Geometry: final body of the model. Coordinates: model frame, mm. A direction names the side the tool comes from. Give positions to 0.01 mm unless a question says otherwise; leave off trailing zeros. Write each loop counter-clockwise with the first axis right and the second up, starting at its lowest first coordinate (ties: lowest second). Pieces come first, ordered by that corner, then holes. Notation, with made-up numbers: M -1.5,-14.75 L 33.5,-14.75 A17 ccw 33.5,17.25 Z; hole C 71.25,2 d10. An arc over 180 degrees is marked long. Use a Markdown table: item, result. Add a question column.
(1) Cut plane C-C (z = 20). Output: boundary loops of the cut face in (x, y) (3 decimals), plus the area to 3 significant figures.
(2) Cut plane A-A (y = -39.5). Output: boundary loops of the cut face in (x, z) (3 decimals).
(3) Cut plane D-D (z = 63). Output: boundary loops of the cut face in (x, y) (3 decimals), plus the area to 3 significant figures.
(4) Material intervals for L1, parallel to X at y = -28.5, z = 153 (3 decimals); L2, parallel to Y at x = -20.25, z = 102.5 (3 decimals); L3, parallel to Y at x = -13.5, z = 16.5 (3 decimals), sorted ascending.
(5) Reachability of faces 1 (the flat face through (0, -20, 100)), 2 (the flat face through (-22.225, -26, 100)) from +Z, -Z, +X, -X, +Y, -Y: full face, straight path, thin tool, end or side. Return the list, or none.
(6) Pin query (flat end, axial travel): pin 1 Ø12 at (x, y) = (-11.5, -41.5) entering from -Z; pin 2 Ø10 at (x, y) = (-19.5, -17.5) entering from -Z. Return the tip coordinate at first contact, or that it passes through.
(7) Cut plane B-B (x = -18.5). Output: boundary loops of the cut face in (y, z) (3 decimals).
Autodesk Inventor part; units mm, degrees
ref_plane "YZ Plane" through (0, 0, 0) normal (1, 0, 0) x (0, 1, 0)
ref_plane "XZ Plane" through (0, 0, 0) normal (0, 1, 0) x (-1, 0, 0)
ref_plane "XY Plane" through (0, 0, 0) normal (0, 0, 1) x (1, 0, 0)
sketch "Sketch1" plane through (0, 0, 0) normal (0, 0, 1) x (1, 0, 0)
  line L0 (0, 0) -> (-25.4, 0)
  line L1 (-25.4, 0) -> (-25.4, -50.8)
  line L2 (-25.4, -50.8) -> (0, -50.8)
  line L3 (0, -50.8) -> (0, 0)
  line L4 (-22.225, -3.175) -> (-3.175, -3.175)
  line L5 (-3.175, -3.175) -> (-3.175, -47.625)
  line L6 (-3.175, -47.625) -> (-22.225, -47.625)
  line L7 (-22.225, -47.625) -> (-22.225, -3.175)
  dimension "d0" = 25.4
  dimension "d1" = 50.8
  dimension "d2" = 3.175
extrude "Extrusion1" add sketch "Sketch1" along normal blind 203.2
sketch "Sketch2" plane through (0, -50.8, 0) normal (1, 0, 0) x (0, 0, -1)
  line L0 (-203.2, 50.8) -> (-152.4, 0)
  line L1 (0, 0) -> (-203.2, 0)
  line L2 (-203.2, 0) -> (-152.4, 0)
  line L3 (-203.2, 0) -> (-203.2, 50.8)
  line L4 (0, 50.8) -> (0, 0)
  line L5 (0, 50.8) -> (0, 0)
  line L6 (0, 0) -> (-50.8, 0)
  line L7 (0, 50.8) -> (-50.8, 0)
  dimension "d5" = 45
  dimension "d6" = 45
  dimension "d7" = 90
  dimension "d8" = 71.8421
  dimension "d9" = 50.8
  dimension "d10" = 50.8
  dimension "d11" = 45
  dimension "d12" = 45
  dimension "d13" = 71.8421
extrude "Extrusion2" cut sketch "Sketch2" against normal blind 203.2
properties part number "Arm Angle brace"
Answer list:
| question | item | result |
|---|---|---|
| 1 | outline | M -25.4,-20 L -22.225,-20 L -22.225,-3.175 L -3.175,-3.175 L -3.175,-20 L 0,-20 L 0,0 L -25.4,0 Z |
| 1 | area | 187 mm² |
| 2 | outline | M -25.4,39.5 L -22.225,39.5 L -22.225,163.7 L -25.4,163.7 Z; M -3.175,39.5 L 0,39.5 L 0,163.7 L -3.175,163.7 Z |
| 3 | outline | M -25.4,-50.8 L 0,-50.8 L 0,0 L -25.4,0 Z; hole M -22.225,-47.625 L -3.175,-47.625 L -3.175,-3.175 L -22.225,-3.175 Z |
| 3 | area | 444 mm² |
| 4 | L1 | -25.4 to -22.225, -3.175 to 0 |
| 4 | L2 | -50.8 to -47.625, -3.175 to 0 |
| 4 | L3 | -3.175 to 0 |
| 5 | face 1 | +Z, -Z, +X, +Y, -Y |
| 5 | face 2 | +Z, -Z |
| 6 | pin 1 | through |
| 6 | pin 2 | z = 13.31 |
| 7 | outline | M -50.8,50.8 L -47.625,47.625 L -47.625,155.575 L -50.8,152.4 Z; M -3.175,3.175 L 0,0 L 0,203.2 L -3.175,200.025 Z |
